Read the model definition and answer for the solid it produces. Units are mm, in the model's axes. Face numbers are marked on the shaded views. A direction names the side the tool comes from. Round coordinates to 2 decimals unless told otherwise and drop trailing zeros. Loops run counter-clockwise (first coordinate to the right, second up) from the corner with the lowest first, then second, coordinate; pieces in that order, holes last. Notation, with made-up numbers: M 51.5,87 L 85.5,87 A24 cw 85.5,113 Z; hole C 42.25,2 d7. An arc over 180 degrees is marked long. Write each question's results on one line, items separated by ' | '.
from build123d import *

# Parameters (mm, degrees)
SKETCH1_R         = 2
EXTRUDE_311_DEPTH = 45
EXTRUDE_445_DEPTH = 4
CHAMFER1_SIZE     = 1


with BuildPart() as part:
    # Sketch1 → Extrude 311 (new body)
    with BuildSketch(Plane.XY):
        with Locations(Location((0, 0, 0), (0, 0, 180))):
            Circle(SKETCH1_R)
    extrude(amount=EXTRUDE_311_DEPTH)

    # Sketch2 → Extrude 445 (add)
    with BuildSketch(Plane.XY.offset(45)):
        Polygon((0, 4.041451884), (-3.5, 2.020725942), (-3.5, -2.020725942), (0, -4.041451884), (3.5, -2.020725942), (3.5, 2.020725942), align=None)
    extrude(amount=EXTRUDE_445_DEPTH)

    # Chamfer1
    chamfer1_edges = [part.edges().sort_by_distance(p)[0] for p in [
        (2, 0, 0),
    ]]
    chamfer(chamfer1_edges, length=CHAMFER1_SIZE)


solid = part.part
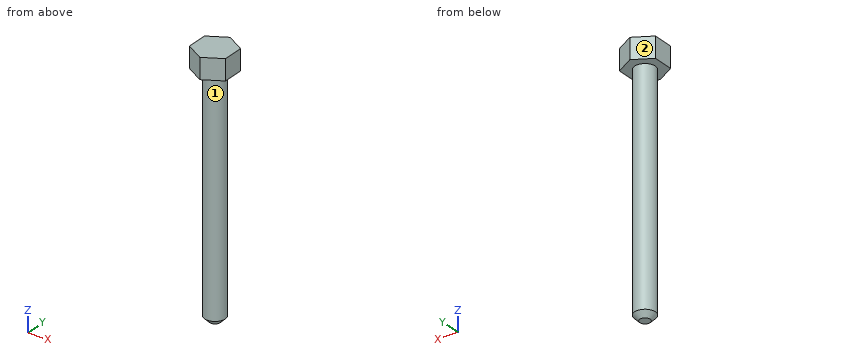
Item 1: For the marked faces 1 and 2, determine the directions among +Z, -Z, +X, -X, +Y, -Y from which every point of the face is accessible in a straight line to the end or side of a thin tool.
Outcome:
face 1: -Z | face 2: +Z, -Z, -X, +Y
Item 2: Flat-ended cylindrical pins translate along their axes: pin 1 (1.5 mm diameter, centred on y = -1.5, z = 36.5, fed in from -X); pin 2 (1.5 mm diameter, centred on x = 0.5, z = 22, fed in from +Y); pin 3 (3.5 mm diameter, centred on x = -1.5, y = 0, fed in from -Z); pin 4 (2 mm diameter, centred on x = 0, y = 2.5, fed in from -Z). Find the tip coordinate at first contact, or state that the pin passes through.
Outcome:
pin 1: stops at x = -1.85 | pin 2: stops at y = 2 | pin 3: stops at z = 0 | pin 4: stops at z = 0.5
Item 3: The part is cut by section A-A (y = 0). Determine the outline of the cut face in (x, z).
Outcome:
outline: M -3.5,45 L -2,45 L -2,1 L -1,0 L 1,0 L 2,1 L 2,45 L 3.5,45 L 3.5,49 L -3.5,49 Z
Item 4: Straight lines are drawn through the part: line 1 (Z direction, x = 2, y = 2.5); line 2 (X direction, y = -1.25, z = 25); line 3 (Y direction, x = -1.5, z = 29). For each, find the intervals that lie inside material, in ascending order.
Outcome:
line 1: z = 45 to 49 | line 2: x = -1.56 to 1.56 | line 3: y = -1.32 to 1.32
Item 5: The part is cut by section B-B (z = 32). Determine the outline of the cut face in (x, y), plus the area to 3 significant figures.
Outcome:
outline: C 0,0 d4 | area: 12.6 mm2
